Work out the finished part from the listing and answer in its coordinate system (mm). A direction names the side the tool comes from. Round coordinates to 2 decimals unless told otherwise and drop trailing zeros. Order: outer loops, then holes, each group sorted by start corner. A loop starts at its lowest first (then second) coordinate and runs counter-clockwise, first axis right, second up. Notation, with made-up numbers: (-30, -7.75) - (-17, -7.75) arc R11 cw to (-17, 12.25) - close; hole circle Ø5 at (-23.5, 86). An arc over 180 degrees is marked (long way). Answer in a Markdown table with one row per item.
from build123d import *

# Parameters (mm, degrees)
SKETCH1_R           = 2.0701
BOSS_EXTRUDE1_DEPTH = 2.286


with BuildPart() as part:
    # Sketch1 → Boss-Extrude1 (new body)
    with BuildSketch(Plane.XY.offset(2.286)):
        with BuildLine():
            Line((16.688088175, 54.0506166), (-12.014209682, 4.336778419))
            Line((-12.014209682, 4.336778419), (-12.573, 2.25134456))
            Line((-12.573, 2.25134456), (-12.573, -55.153251153))
            Line((-12.573, -55.153251153), (-11.4935, -57.023))
            Line((-11.4935, -57.023), (10.703251153, -57.023))
            Line((10.703251153, -57.023), (12.573, -55.9435))
            Line((12.573, -55.9435), (12.573, -5.070402568))
            ThreePointArc((12.573, -5.070402568), (12.789371003, -3.426901632), (13.423738686, -1.895402568))
            Line((13.423738686, -1.895402568), (38.860287402, 42.161992177))
            Line((38.860287402, 42.161992177), (37.780787402, 44.031741023))
            Line((37.780787402, 44.031741023), (18.557837022, 55.1301166))
            Line((18.557837022, 55.1301166), (16.688088175, 54.0506166))
        make_face()
        Circle(SKETCH1_R, mode=Mode.SUBTRACT)
        with Locations((0, -38.1)):
            Circle(SKETCH1_R, mode=Mode.SUBTRACT)
        with Locations((0, -12.7)):
            Circle(SKETCH1_R, mode=Mode.SUBTRACT)
        with Locations((0, -25.4)):
            Circle(SKETCH1_R, mode=Mode.SUBTRACT)
        with Locations((0, -50.8)):
            Circle(SKETCH1_R, mode=Mode.SUBTRACT)
        with Locations((19.05, 32.995567884)):
            Circle(SKETCH1_R, mode=Mode.SUBTRACT)
        with Locations((6.35, 10.998522628)):
            Circle(SKETCH1_R, mode=Mode.SUBTRACT)
        with Locations((12.7, 21.997045256)):
            Circle(SKETCH1_R, mode=Mode.SUBTRACT)
        with Locations((25.4, 43.994090512)):
            Circle(SKETCH1_R, mode=Mode.SUBTRACT)
    extrude(amount=-BOSS_EXTRUDE1_DEPTH)


solid = part.part
1) This flat-tipped pin is pushed along its axis until it touches: pin 1 (0.7 mm diameter, centred on y = -40, z = 1, fed in from +X). Where does it stop, or does it pass through?
Filled in:
| item | result |
|---|---|
| pin 1 | stops at x = 12.57 |
2) Find section B-B, the plane x = 6.5. Give the vertices of the cut face in (y, z), then the cut area to 3 significant figures.
Filled in:
| item | result |
|---|---|
| outline | (-57.02, 0) - (8.93, 0) - (8.93, 2.29) - (-57.02, 2.29) - close; (13.06, 0) - (36.4, 0) - (36.4, 2.29) - (13.06, 2.29) - close |
| area | 204 mm^2 |
3) Find section D-D, the plane y = 25.5. Give the vertices of the cut face in (x, z), then the cut area to 3 significant figures.
Filled in:
| item | result |
|---|---|
| outline | (0.2, 0) - (29.24, 0) - (29.24, 2.29) - (0.2, 2.29) - close |
| area | 66.4 mm^2 |
4) Find the intervals of material crossed by probe 1 along Y at (x, z) = (0, 1.25); probe 2 along Y at (x, z) = (0.5, 0.2); probe 3 along X at (y, z) = (-36, 1.1), in increasing order. Write a range as from..to.
Filled in:
| item | result |
|---|---|
| probe 1 | y = -57.02..-52.87, -48.73..-40.17, -36.03..-27.47, -23.33..-14.77, -10.63..-2.07, 2.07..25.15 |
| probe 2 | y = -57.02..-52.81, -48.79..-40.11, -36.09..-27.41, -23.39..-14.71, -10.69..-2.01, 2.01..26.01 |
| probe 3 | x = -12.57..12.57 |
5) Which of the six approach directions +Z, -Z, +X, -X, +Y, -Y give full straight-line access (tool end or side, diameter ignored) to faces 1 (the face through (7, 0, 0)), 2 (the face through (12.573, -31, 1))?
Filled in:
| item | result |
|---|---|
| face 1 | -Z, +X, -X, +Y, -Y |
| face 2 | +Z, -Z, +X, -Y |
6) Find section A-A, the plane y = -12.7. Give the vertices of the cut face in (x, z).
Filled in:
| item | result |
|---|---|
| outline | (-12.57, 0) - (-2.07, 0) - (-2.07, 2.29) - (-12.57, 2.29) - close; (2.07, 0) - (12.57, 0) - (12.57, 2.29) - (2.07, 2.29) - close |
7) Find section C-C, the plane z = 0.7. Give the number of separate pieces and of enclosed holes in the cut face, then the cut area to 3 significant figures.
Filled in:
| item | result |
|---|---|
| separate pieces | 1 |
| enclosed holes | 9 |
| area | 2,740 mm^2 |
8) The mould has two halves that part along X. Classify faces 3 (the face through (-0.269, -10.648, 1.159)), 4 (the face through (-12.29, 3.31, 1.16)), 5 (the face through (12.783, -3.449, 1.159)), 6 (the face through (-0.269, -36.048, 1.159)): released by +X, released by -X, zero draft, split by the parting line, or undercut.
Filled in:
| item | result |
|---|---|
| face 3 | undercut |
| face 4 | released by -X |
| face 5 | released by +X |
| face 6 | undercut |
